from build123d import *

# Parameters (mm, degrees)
SKETCH1_W           = 67.749
SKETCH1_H           = 25.656
BOSS_EXTRUDE1_DEPTH = 7.9375
SKETCH2_R           = 3
BOSS_EXTRUDE2_DEPTH = 144.4625
BOSS_EXTRUDE4_DEPTH = 8.448


with BuildPart() as part:
    # Sketch1 → Boss-Extrude1 (new body)
    with BuildSketch(Plane(origin=(0, 0, 0), x_dir=(1, 0, 0), z_dir=(0, 1, 0))):
        Rectangle(SKETCH1_W, SKETCH1_H)
    extrude(amount=BOSS_EXTRUDE1_DEPTH)

    # Sketch2 → Boss-Extrude2 (add)
    with BuildSketch(Plane(origin=(0, 7.9375, 0), x_dir=(1, 0, 0), z_dir=(0, 1, 0))):
        with Locations(Location((26.2085, 0, 0), (0, 0, 90))):
            Circle(SKETCH2_R)
    extrude(amount=BOSS_EXTRUDE2_DEPTH)

    # Sketch3 → Boss-Extrude4 (add)
    with BuildSketch(Plane.XZ):
        Polygon((22.0835, -7.144709581), (30.3335, -7.144709581), (34.4585, 0), (30.3335, 7.144709581), (22.0835, 7.144709581), (17.9585, 0), align=None)
    extrude(amount=BOSS_EXTRUDE4_DEPTH)


solid = part.part
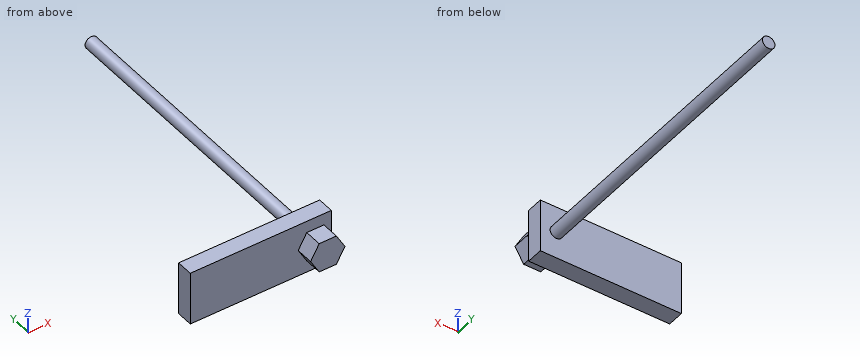
Could you check a few things on this model? Use its own coordinates, in mm. Coordinates: 2 decimals unless noted, no trailing zeros. Order: outer loops, then holes, each group sorted by start corner. A loop starts at its lowest first (then second) coordinate and runs counter-clockwise, first axis right, second up. Notation, with made-up numbers: (-39, -39.75) -> (9, -39.75) arc R29 ccw to (9, -14.75) -> close; hole circle Ø7 at (-8, -14.5). An arc over 180 degrees is marked (long way). One line per item, written item: value. Start each with the question number.
1) Imagine slicing it at B-B on x = 6. List the corners of the cut face in (y, z) for me, plus the area to 3 significant figures.
2) I'm going to push flat-ended pins straight in: pin 1 (6.5 mm diameter, centred on x = 26.5, y = -4.5, fed in from -Z); pin 2 (10 mm diameter, centred on y = 77, z = -3, fed in from -X); pin 3 (2.5 mm diameter, centred on y = 3, z = 6, fed in from +X). Where does each tip first touch, or does it pass through?
3) Imagine slicing it at C-C on y = 74. List the corners of the cut face in (x, z) for me, plus the area to 3 significant figures.
4) Imagine slicing it at A-A on z = -4.5. List the corners of the cut face in (x, y) for me, plus the area to 3 significant figures.
5) If I drill on L1, parallel to Y at x = 2, z = 9.5; L2, parallel to Y at x = 22, z = -5.25; L3, parallel to X at y = 7, z = 0, over which ranges is the centre line in solid material (lowest first)? Write a range as [from, to].
Answer list:
1. outline: (0, -12.83) -> (7.94, -12.83) -> (7.94, 12.83) -> (0, 12.83) -> close
1. area: 204 mm2
2. pin 1: stops at z = -7.14
2. pin 2: stops at x = 23.21
2. pin 3: stops at x = 33.87
3. outline: circle Ø6 at (26.21, 0)
3. area: 28.3 mm2
4. outline: (-33.87, 0) -> (20.56, 0) -> (20.56, -8.45) -> (31.86, -8.45) -> (31.86, 0) -> (33.87, 0) -> (33.87, 7.94) -> (-33.87, 7.94) -> close
4. area: 633 mm2
5. L1: y = [0, 7.94]
5. L2: y = [-8.45, 7.94]
5. L3: x = [-33.87, 33.87]
